```python
from build123d import *

# Parameters (mm, degrees)
ESQUISSE1_R        = 1.5
BOSS_EXTRU_1_DEPTH = 3
ESQUISSE2_R        = 6
ESQUISSE2_R_2      = 4.5
BOSS_EXTRU_2_DEPTH = 15
CONG_1_R           = 0.5


with BuildPart() as part:
    # Esquisse1 → Boss.-Extru.1 (new body)
    with BuildSketch(Plane.XY):
        with BuildLine():
            Line((7.5, -12.5), (-7.5, -12.5))
            ThreePointArc((-7.5, -12.5), (-11.035533906, -11.035533906), (-12.5, -7.5))
            Line((-12.5, -7.5), (-12.5, 7.5))
            ThreePointArc((-12.5, 7.5), (-11.035533906, 11.035533906), (-7.5, 12.5))
            Line((-7.5, 12.5), (7.5, 12.5))
            ThreePointArc((7.5, 12.5), (11.035533906, 11.035533906), (12.5, 7.5))
            Line((12.5, 7.5), (12.5, -7.5))
            ThreePointArc((12.5, -7.5), (11.035533906, -11.035533906), (7.5, -12.5))
        make_face()
        with Locations((-7.5, 7.5)):
            Circle(ESQUISSE1_R, mode=Mode.SUBTRACT)
        with Locations((7.5, 7.5)):
            Circle(ESQUISSE1_R, mode=Mode.SUBTRACT)
        with Locations((7.5, -7.5)):
            Circle(ESQUISSE1_R, mode=Mode.SUBTRACT)
        with Locations((-7.5, -7.5)):
            Circle(ESQUISSE1_R, mode=Mode.SUBTRACT)
    extrude(amount=BOSS_EXTRU_1_DEPTH)

    # Esquisse2 → Boss.-Extru.2 (add)
    with BuildSketch(Plane.XY.offset(3)):
        Circle(ESQUISSE2_R)
        Circle(ESQUISSE2_R_2, mode=Mode.SUBTRACT)
    extrude(amount=BOSS_EXTRU_2_DEPTH)

    # Congé1
    cong_1_edges = [part.edges().sort_by_distance(p)[0] for p in [
        (-6, 0, 18),
        (-6, 0, 3),
        (-4.5, 0, 18),
    ]]
    fillet(cong_1_edges, radius=CONG_1_R)


solid = part.part
```
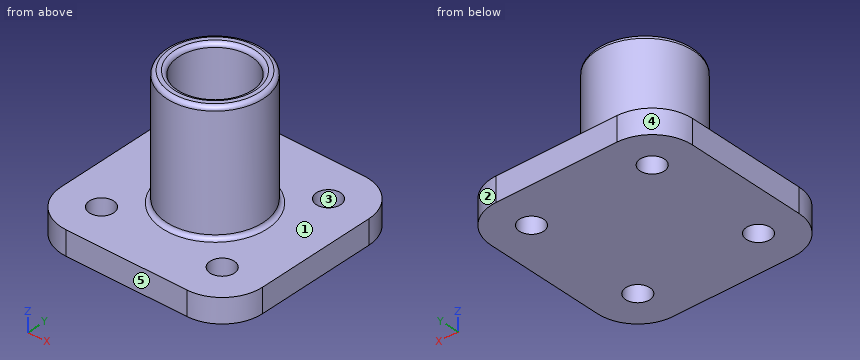
Input: part model. Units: mm. Frame: model coordinates. Face numbers are marked on the shaded views. A direction names the side the tool comes from. Round coordinates to 2 decimals unless told otherwise and drop trailing zeros. Loops run counter-clockwise (first coordinate to the right, second up) from the corner with the lowest first, then second, coordinate; pieces in that order, holes last. Notation, with made-up numbers: M -34,-39 L 20,-39 A20 ccw 20,-5 Z; hole C -26,-5.5 d6. An arc over 180 degrees is marked long. Answer in a Markdown table with one row per item. Add a question column.
1. Section D-D (z = 7.25). Output: boundary loops of the cut face in (x, y), and give its area (3 significant figures).
2. Section C-C (y = 0). Output: boundary loops of the cut face in (x, z).
3. Section A-A (z = 1.75). Output: boundary loops of the cut face in (x, y).
4. Set-up query: the marked faces 1 and 2. Return all of +Z, -Z, +X, -X, +Y, -Y with unobstructed straight access to the full face (end or side cutting, diameter ignored); none if empty.
5. Section B-B (x = -8.5). Output: boundary loops of the cut face in (y, z), and give its area (3 significant figures).
6. Ray query, probe 1 along Y at (x, z) = (-7.5, 1.95); probe 2 along Y at (x, z) = (0, 6); probe 3 along Z at (x, y) = (-8.5, -4). Return the intervals inside material, ascending.
7. Contact query for flat-ended pins moving along their axis: pin 1 (5 mm diameter, centred on x = -5, y = -1, fed in from -Z); pin 2 (2 mm diameter, centred on x = -1.5, y = 2, fed in from +Z); pin 3 (5 mm diameter, centred on y = -2.5, z = 15, fed in from +X); pin 4 (3 mm diameter, centred on x = -4, z = 8, fed in from -Y). Output: stop coordinate, or through.
8. Mould query, pull axis X, two halves, no side actions, for the marked faces 3, 4 and 5. Classes: released by +X, released by -X, zero draft, split by the parting line, or undercut.
Values follow:
| question | item | result |
|---|---|---|
| 1 | outline | C 0,0 d12; hole C 0,0 d9 |
| 1 | area | 49.5 mm^2 |
| 2 | outline | M -12.5,0 L 12.5,0 L 12.5,3 L 6.5,3 A0.5 cw 6,3.5 L 6,17.5 A0.5 ccw 5.5,18 L 5,18 A0.5 ccw 4.5,17.5 L 4.5,3 L -4.5,3 L -4.5,17.5 A0.5 ccw -5,18 L -5.5,18 A0.5 ccw -6,17.5 L -6,3.5 A0.5 cw -6.5,3 L -12.5,3 Z |
| 3 | outline | M -12.5,-7.5 A5 ccw -7.5,-12.5 L 7.5,-12.5 A5 ccw 12.5,-7.5 L 12.5,7.5 A5 ccw 7.5,12.5 L -7.5,12.5 A5 ccw -12.5,7.5 Z; hole C -7.5,-7.5 d3; hole C -7.5,7.5 d3; hole C 7.5,-7.5 d3; hole C 7.5,7.5 d3 |
| 4 | face 1 | +Z |
| 4 | face 2 | +Z, -Z, +X, +Y |
| 5 | outline | M -12.4,0 L -8.62,0 L -8.62,3 L -12.4,3 Z; M -6.38,0 L 6.38,0 L 6.38,3 L -6.38,3 Z; M 8.62,0 L 12.4,0 L 12.4,3 L 8.62,3 Z |
| 5 | area | 61.0 mm^2 |
| 6 | probe 1 | -12.5 to -9, -6 to 6, 9 to 12.5 |
| 6 | probe 2 | -6 to -4.5, 4.5 to 6 |
| 6 | probe 3 | 0 to 3 |
| 7 | pin 1 | z = 0 |
| 7 | pin 2 | z = 3 |
| 7 | pin 3 | x = 6 |
| 7 | pin 4 | y = -5.45 |
| 8 | face 3 | undercut |
| 8 | face 4 | released by -X |
| 8 | face 5 | zero draft |
